Read the model definition and answer for the solid it produces. Units are mm, in the model's axes. Face numbers are marked on the shaded views. Give positions to 0.01 mm unless a question says otherwise; leave off trailing zeros. Order: outer loops, then holes, each group sorted by start corner. A loop starts at its lowest first (then second) coordinate and runs counter-clockwise, first axis right, second up.
Item 1: The mould has two halves that part along Z. Classify the marked faces 1, 2 and 3: +Z half, -Z half, draft (parallel to the pull), parting line (faces both ways), or undercut.
Item 2: A cutting plane is placed at C-C (z = 1). Write down the section's boundary in (x, y), plus the area to 3 significant figures.
Item 3: A cutting plane is placed at B-B (x = 24). Write down the section's boundary in (y, z).
Item 4: A cutting plane is placed at A-A (y = 7.75). Write down the section's boundary in (x, z), plus the area to 3 significant figures.
Item 5: Given pin 1 Ø1.6 at (y, z) = (13.5, 8.5) entering from -X; pin 2 Ø2 at (y, z) = (7.75, 7.75) entering from +X; pin 3 Ø3 at (x, y) = (22.5, 14.5) entering from +Z; pin 4 Ø2.5 at (y, z) = (1.5, 10.5) entering from -X, each flat-ended and moving along its own axis, determine where each tip first touches the part or whether it passes through.
Item 6: Find the intervals of material crossed by line 1 along X through (y, z) = (6, 3.75); line 2 along Y through (x, z) = (52, 7.75); line 3 along Y through (x, z) = (6.5, 5), in increasing order.
from build123d import *

# Parameters (mm, degrees)
F0_W         = 49
F0_H         = 15.5
F1_DEPTH     = 2.5
F3_DEPTH     = 49
F4_R         = 1
F5_R         = 5
F7_DEPTH     = 10
F9_DEPTH     = 10
F10_W        = 10
F10_H        = 6.7160013448
F10_W_2      = 9
F11_DEPTH    = 15.501
F12_T1_DEPTH = 36.7168298797
F12_T3_DEPTH = 33.4668298797
F13_R        = 1.25
F14_DEPTH    = 69.001
F15_W        = 1
F15_H        = 2
F16_DEPTH    = 15.501
F17_R        = 3.15
F18_DEPTH    = 1


# Not quite as in the source:
# - a fillet or chamfer that OpenCascade refuses, or shapes differently, is made with other operations: its cross-section is extruded or revolved along the edge and cut away or added


with BuildPart() as f1:
    # F0 (on Top) → F1 (new body)
    with BuildSketch(Plane.XY):
        with Locations((24.5, 7.75)):
            Rectangle(F0_W, F0_H)
    extrude(amount=F1_DEPTH)

    # F2 (on Right) → F3 (join, through all)
    with BuildSketch(Plane.YZ):
        with BuildLine():
            Line((0, 7.75), (0, 2.5))
            Line((0, 2.5), (2.5, 2.5))
            Line((2.5, 2.5), (2.5, 7.75))
            ThreePointArc((2.5, 7.75), (2.690862635, 9.1752192814), (3.25, 10.5))
            Line((3.25, 10.5), (3.25, 14.1449850143))
            ThreePointArc((3.25, 14.1449850143), (0.859115549, 11.3367232028), (0, 7.75))
        make_face()
        with BuildLine():
            Line((13, 7.75), (13, 2.5))
            Line((13, 2.5), (15.5, 2.5))
            Line((15.5, 2.5), (15.5, 7.75))
            ThreePointArc((15.5, 7.75), (14.640884451, 11.3367232028), (12.25, 14.1449850143))
            Line((12.25, 14.1449850143), (12.25, 10.5))
            ThreePointArc((12.25, 10.5), (12.809137365, 9.1752192814), (13, 7.75))
        make_face()
    extrude(amount=F3_DEPTH)

    # F4
    f4_edges = [f1.edges().sort_by_distance(p)[0] for p in [
        (24.5, 12.25, 14.144985),
        (24.5, 3.25, 14.144985),
    ]]
    fillet(f4_edges, radius=F4_R)

    # F5
    f5_edges = [f1.edges().sort_by_distance(p)[0] for p in [
        (24.5, 12.25, 10.5),
        (24.5, 3.25, 10.5),
    ]]
    fillet(f5_edges, radius=F5_R)

    # F6 (on face) → F7 (join)
    with BuildSketch(Plane(origin=(0, 0, 0), x_dir=(0, -1, 0), z_dir=(-1, 0, 0))):
        with BuildLine():
            ThreePointArc((-14.0692771084, 12.2893991295), (-15.1338520571, 10.1297642977), (-15.5, 7.75))
            Line((-15.5, 7.75), (-15.5, 0))
            Line((-15.5, 0), (0, 0))
            Line((0, 0), (0, 7.75))
            ThreePointArc((0, 7.75), (-0.3661479429, 10.1297642977), (-1.4307228916, 12.2893991295))
            ThreePointArc((-1.4307228916, 12.2893991295), (-1.7881546713, 12.6029618244), (-2.25, 12.7160013448))
            Line((-2.25, 12.7160013448), (-13.25, 12.7160013448))
            ThreePointArc((-13.25, 12.7160013448), (-13.7118453287, 12.6029618244), (-14.0692771084, 12.2893991295))
        make_face()
    extrude(amount=F7_DEPTH)

    # F8 (on face) → F9 (join)
    with BuildSketch(Plane.YZ.offset(49)):
        with BuildLine():
            Line((15.5, 0), (15.5, 7.75))
            ThreePointArc((15.5, 7.75), (15.1338520571, 10.1297642977), (14.0692771084, 12.2893991295))
            ThreePointArc((14.0692771084, 12.2893991295), (13.7118453287, 12.6029618244), (13.25, 12.7160013448))
            Line((13.25, 12.7160013448), (2.25, 12.7160013448))
            ThreePointArc((2.25, 12.7160013448), (1.7881546713, 12.6029618244), (1.4307228916, 12.2893991295))
            ThreePointArc((1.4307228916, 12.2893991295), (0.3661479429, 10.1297642977), (0, 7.75))
            Line((0, 7.75), (0, 0))
            Line((0, 0), (15.5, 0))
        make_face()
    extrude(amount=F9_DEPTH)

    # F10 (on face) → F11 (cut, through all)
    with BuildSketch(Plane.XZ):
        with Locations((44, 9.3580006724)):
            Rectangle(F10_W, F10_H)
        with Locations((24.5, 9.3580006724)):
            Rectangle(F10_W_2, F10_H)
        with Locations((5, 9.3580006724)):
            Rectangle(F10_W, F10_H)
    extrude(amount=-F11_DEPTH, mode=Mode.SUBTRACT)

    # F12: chamfer of 5 on 6 edges, made by hand

    # F12_s2 → F12_t1 (cut)
    with BuildSketch(Plane.XZ.offset(-26.1084149398)):
        Polygon((-10, 7.7160013448), (-5, 12.7160013448), (-10, 12.7160013448), align=None)
        Polygon((54, 12.7160013448), (59, 7.7160013448), (59, 12.7160013448), align=None)
    extrude(amount=F12_T1_DEPTH, mode=Mode.SUBTRACT)

    # F12_s4 → F12_t3 (cut)
    with BuildSketch(Plane.XY.offset(-12.8584149398)):
        Polygon((-10, 5), (-5, 0), (-10, 0), align=None)
        Polygon((-5, 15.5), (-10, 10.5), (-10, 15.5), align=None)
        Polygon((54, 0), (59, 5), (59, 0), align=None)
        Polygon((54, 15.5), (59, 10.5), (59, 15.5), align=None)
    extrude(amount=F12_T3_DEPTH, mode=Mode.SUBTRACT)

    # F13 (on face) → F14 (cut, through all)
    with BuildSketch(Plane(origin=(-10, 0, 0), x_dir=(0, -1, 0), z_dir=(-1, 0, 0))):
        with Locations((-7.75, 7.75)):
            Circle(F13_R)
    extrude(amount=-F14_DEPTH, mode=Mode.SUBTRACT)

    # F15 (on face) → F16 (cut, through all)
    with BuildSketch(Plane.XZ):
        with Locations((48.5, 3.5)):
            Rectangle(F15_W, F15_H)
    extrude(amount=-F16_DEPTH, mode=Mode.SUBTRACT)

    # F17 (on face) → F18 (cut)
    with BuildSketch(Plane(origin=(49, 0, 0), x_dir=(0, -1, 0), z_dir=(-1, 0, 0))):
        with Locations((-7.75, 7.75)):
            Circle(F17_R)
    extrude(amount=-F18_DEPTH, mode=Mode.SUBTRACT)


solid = f1.part
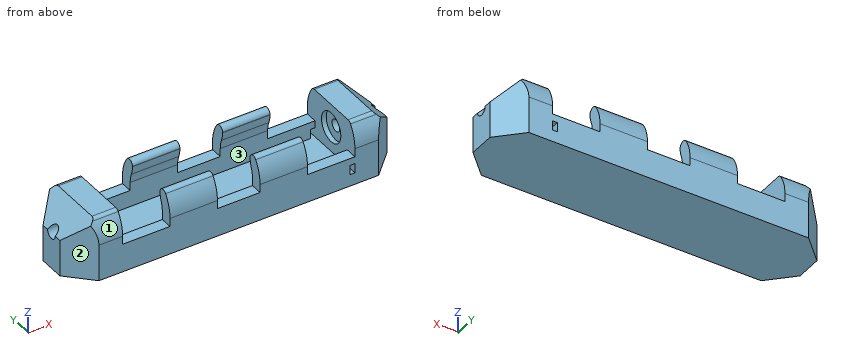
Response values:
1. face 1: +Z half
1. face 2: draft
1. face 3: undercut
2. outline: (-10, 5) - (-5, 0) - (54, 0) - (59, 5) - (59, 10.5) - (54, 15.5) - (-5, 15.5) - (-10, 10.5) - close
2. area: 1,020 mm2
3. outline: (0, 0) - (15.5, 0) - (15.5, 6) - (13, 6) - (13, 2.5) - (2.5, 2.5) - (2.5, 6) - (0, 6) - close
4. outline: (-10, 0) - (59, 0) - (59, 6.5) - (50, 6.5) - (50, 4.6) - (49, 4.6) - (49, 2.5) - (0, 2.5) - (0, 6.5) - (-10, 6.5) - close; (-8.72, 9) - (0, 9) - (0, 12.72) - (-5, 12.72) - close; (49, 10.9) - (50, 10.9) - (50, 9) - (57.72, 9) - (54, 12.72) - (49, 12.72) - close
4. area: 300 mm2
5. pin 1: stops at x = -7.8
5. pin 2: passes through
5. pin 3: stops at z = 6
5. pin 4: stops at x = -7.67
6. line 1: x = -10 to 0, 49 to 59
6. line 2: y = 0 to 6.5, 9 to 15.5
6. line 3: y = 0 to 2.5, 13 to 15.5
